Work out the finished part from the listing and answer in its coordinate system (mm). Face numbers are marked on the shaded views. Give positions to 0.01 mm unless a question says otherwise; leave off trailing zeros. Loops run counter-clockwise (first coordinate to the right, second up) from the corner with the lowest first, then second, coordinate; pieces in that order, holes last. Notation, with made-up numbers: (36.25, 79.5) -> (51.25, 79.5) arc R20 cw to (51.25, 86.5) -> close; hole circle Ø10 at (40.25, 65.25). An arc over 180 degrees is marked (long way). Answer as CSV lines item,"result". Start each with the question number.
1. Determine the mould class of the marked faces 1, 2, 3 and 4 for opening direction Y: +Y half, -Y half, draft (parallel to the pull), parting line (faces both ways), or undercut.
2. Find section D-D, the plane z = 1.25. Give the vertices of the cut face in (x, y) (1 decimal), and give its area (3 significant figures).
3. Flat-ended cylindrical pins translate along their axes: pin 1 Ø2 at (x, z) = (2.5, 2.5) entering from -Y; pin 2 Ø3 at (x, y) = (-1.5, 1.5) entering from -Z; pin 3 Ø1.5 at (y, z) = (-3, -2) entering from +X; pin 4 Ø2 at (y, z) = (-1.5, -6) entering from -X. Find the tip coordinate at first contact, or state that the pin passes through.
4. Find the intervals of material crossed by line 1 along Z through (x, y) = (3.9, 0); line 2 along X through (y, z) = (1.5, -0.5); line 3 along X through (y, z) = (-3, -1.25), in increasing order.
5. Find section B-B, the plane z = -3.95. Give the vertices of the cut face in (x, y) (1 decimal), and give its area (3 significant figures).
6. Find section C-C, the plane z = -1.75. Give the vertices of the cut face in (x, y) (1 decimal), and give its area (3 significant figures).
7. Find section A-A, the plane y = 0. Count the separate pieces of the cut face and the enclosed holes in it, and give its area (3 significant figures).
from build123d import *

# Parameters (mm, degrees)
SKETCH1_R                = 4.1275
BOSS_EXTRUDE1_DEPTH      = 6.35
BOSS_EXTRUDE1_DEPTH_BACK = 7.62
CUT_EXTRUDE1_DEPTH       = 7.874
F_2_CLEARANCE_HOLE1_D    = 2.7051
CHAMFER1_SIZE            = 0.508


with BuildPart() as part:
    # Sketch1 → Boss-Extrude1 (new body, two sides)
    with BuildSketch(Plane.XY) as boss_extrude1_sk:
        Circle(SKETCH1_R)
    extrude(amount=BOSS_EXTRUDE1_DEPTH)
    extrude(boss_extrude1_sk.sketch, amount=-BOSS_EXTRUDE1_DEPTH_BACK)

    # Sketch2 → Cut-Extrude1 (cut)
    with BuildSketch(Plane(origin=(0, 0, -7.62), x_dir=(-1, 0, 0), z_dir=(0, 0, -1))):
        with BuildLine():
            Line((-0.746, -3.293929837), (-0.746, 3.293929837))
            ThreePointArc((-0.746, 3.293929837), (-3.377349518, 0), (-0.746, -3.293929837))
        make_face()
        with BuildLine():
            Line((0.746, -3.293929837), (0.746, 3.293929837))
            ThreePointArc((0.746, 3.293929837), (3.377349518, 0), (0.746, -3.293929837))
        make_face()
    extrude(amount=-CUT_EXTRUDE1_DEPTH, mode=Mode.SUBTRACT)

    # #2 Clearance Hole1 (through all)
    with Locations(Plane.ZY.offset(4.1275)):
        with Locations((-3.95, 0)):
            Hole(F_2_CLEARANCE_HOLE1_D / 2)

    # Sketch5 → Hole1 (revolve, cut)
    with BuildSketch(Plane(origin=(0, 0, 6.35), x_dir=(0, -1, 0), z_dir=(1, 0, 0))):
        Polygon((0, 0), (0, 3.81), (2.5273, 3.81), (2.6543, 0), align=None)
    revolve(axis=Axis((0, 0, -103.65), (0, 0, 1)), mode=Mode.SUBTRACT)

    # Chamfer1
    chamfer1_edges = [part.edges().sort_by_distance(p)[0] for p in [
        (3.377349518, 0, -7.62),
        (0.746, 0, -7.62),
        (-3.377349518, 0, -7.62),
        (-0.746, 0, -7.62),
    ]]
    chamfer(chamfer1_edges, length=CHAMFER1_SIZE)


solid = part.part
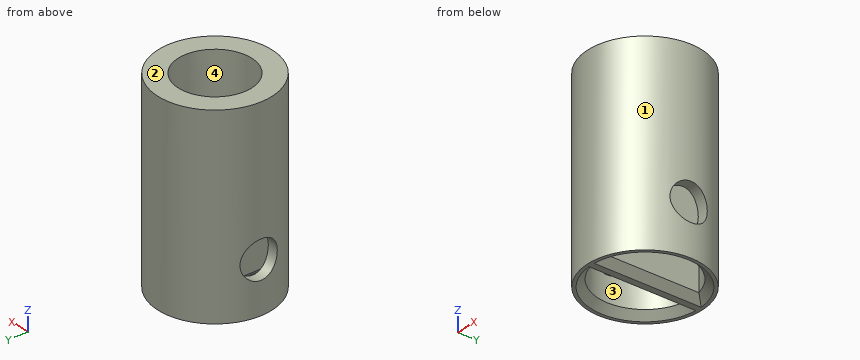
Resolved:
1,face 1,"parting line"
1,face 2,"draft"
1,face 3,"undercut"
1,face 4,"undercut"
2,outline,"circle Ø8.3 at (0, 0)"
2,area,"53.5 mm^2"
3,pin 1,"stops at y = -3.85"
3,pin 2,"stops at z = -7.62"
3,pin 3,"stops at x = 3.46"
3,pin 4,"stops at x = -4.1"
4,line 1,"z = -7.62 to -5.3, -2.6 to 6.35"
4,line 2,"x = -3.85 to -3.03, -0.75 to 0.75, 3.03 to 3.85"
4,line 3,"x = -2.83 to -1.55, -0.75 to 0.75, 1.55 to 2.83"
5,outline,"(-3.9, -1.4) arc R4.1 ccw to (3.9, -1.4) -> (3.1, -1.4) arc R3.4 cw to (0.7, -3.3) -> (0.7, -1.4) -> (-0.7, -1.4) -> (-0.7, -3.3) arc R3.4 cw to (-3.1, -1.4) -> close; (-3.9, 1.4) -> (-3.1, 1.4) arc R3.4 cw to (-0.7, 3.3) -> (-0.7, 1.4) -> (0.7, 1.4) -> (0.7, 3.3) arc R3.4 cw to (3.1, 1.4) -> (3.9, 1.4) arc R4.1 ccw to start"
5,area,"19.5 mm^2"
6,outline,"circle Ø8.3 at (0, 0); hole (-0.7, -3.3) -> (-0.7, 3.3) arc R3.4 ccw to start; hole (0.7, -3.3) arc R3.4 ccw to (0.7, 3.3) -> close"
6,area,"27.7 mm^2"
7,separate pieces,"4"
7,enclosed holes,"0"
7,area,"45.5 mm^2"
